Geometry: final body of the model. Coordinates: model frame, mm. A direction names the side the tool comes from. Give positions to 0.01 mm unless a question says otherwise; leave off trailing zeros. Write each loop counter-clockwise with the first axis right and the second up, starting at its lowest first coordinate (ties: lowest second). Pieces come first, ordered by that corner, then holes.
Autodesk Inventor part; units mm, degrees
ref_plane "Work Plane1" through (4.5, 0, 0) normal (1, 0, 0) x (0, 0, -1)
ref_plane "YZ Plane" through (0, 0, 0) normal (1, 0, 0) x (0, 1, 0)
ref_plane "XZ Plane" through (0, 0, 0) normal (0, 1, 0) x (-1, 0, 0)
sketch "Sketch2" plane through (0, 0, 0) normal (1, 0, 0) x (0, 1, 0)
  line L0 (0, 0) -> (0, -3)
  line L1 (13, 0) -> (13, -16)
  arc A0 (13, 0) -> (0, 0) centre (6.5, 0) ccw
  line L2 (-3.1385, 0) -> (18.8309, 0)
  line L3 (0, -52.4723) -> (0, 16.3287)
  line L4 (0, -3) -> (6.5, -9.5)
  line L5 (0, -3) -> (9.1924, -3) construction
  line L6 (6.5, -9.5) -> (6.5, -16)
  line L7 (6.5, -16) -> (0, -22.5)
  line L8 (6.5, -16) -> (15.6924, -16) construction
  line L9 (0, -22.5) -> (0, -27.5)
  line L10 (0, -27.5) -> (6.5, -34)
  line L11 (0, -27.5) -> (9.1924, -27.5) construction
  line L12 (13, -16) -> (13, -34)
  line L13 (13, -34) -> (13, -40.5)
  arc A1 (6.5, -34) -> (13, -40.5) centre (11.1419, -35.8581) ccw
  circle A2 centre (9.75, -38) radius 1.625
  dimension "d4" = 13
  dimension "d9" = 45
  dimension "d10" = 6.5
  dimension "d11" = 3
  dimension "d12" = 6.5
  dimension "d13" = 135
  dimension "d14" = 6.5
  dimension "d15" = 5
  dimension "d16" = 45
  dimension "d17" = 6.5
  dimension "d18" = 18
  dimension "d19" = 6.5
  dimension "d20" = 5
  dimension "d21" = 3.25
  dimension "d22" = 3.25
  dimension "d23" = 2.5
  dimension "d96" = 16
extrude "Extrusion1" add sketch "Sketch2" along normal mid plane 13 contours L2 L1 L12 L13 A1 L10 L3 L7 L6 L4 L0 | A0 L2
sketch "Sketch3" plane through (-6.5, 13, 0) normal (0, 1, 0) x (1, 0, 0)
  line L0 (0, 34) -> (13, 34)
  line L1 (0, 41) -> (1.5, 41)
  line L2 (1.5, 41) -> (1.5, 34)
  line L3 (1.5, 34) -> (0, 34)
  line L4 (0, 34) -> (0, 41)
  line L5 (0, 0) -> (0, 40.5)
  line L6 (3.5, 41) -> (7.5, 41)
  line L7 (7.5, 41) -> (7.5, 34)
  line L8 (7.5, 34) -> (3.5, 34)
  line L9 (3.5, 34) -> (3.5, 41)
  line L10 (9.5, 41) -> (13, 41)
  line L11 (13, 41) -> (13, 34)
  line L12 (13, 34) -> (9.5, 34)
  line L13 (9.5, 34) -> (9.5, 41)
  line L14 (13, 40.5) -> (13, 0)
  point P0 (6.5, 0)
  dimension "d47" = 1.5
  dimension "d48" = 7
  dimension "d49" = 4
  dimension "d50" = 7
  dimension "d51" = 2
  dimension "d52" = 7
  dimension "d53" = 2
extrude "Extrusion2" cut sketch "Sketch3" against normal blind 13
ref_plane "Work Plane1" through (4.5, 0, 0) normal (1, 0, 0) x (0, 0, -1)
sketch "Sketch4" plane through (4.5, 0, 0) normal (1, 0, 0) x (0, 0, -1)
  arc A0 (0, 13) -> (0, 0) centre (0, 6.5) ccw
  line L0 (0, 13) -> (34, 13)
  line L1 (34, 13) -> (34, 6.5)
  line L2 (34, 6.5) -> (27.5, 0)
  line L3 (27.5, 0) -> (22.5, 0)
  line L4 (22.5, 0) -> (16, 6.5)
  line L5 (34, 13) -> (34, 6.5)
  line L6 (34, 6.5) -> (27.5, 0)
  line L7 (27.5, 0) -> (22.5, 0)
  line L8 (22.5, 0) -> (16, 6.5)
  line L9 (16, 6.5) -> (9.5, 6.5)
  line L10 (9.5, 6.5) -> (3, 0)
  line L11 (3, 0) -> (0, 0)
  arc A1 (0, 13) -> (0, 0) centre (0, 6.5) ccw
  line L12 (0, 13) -> (34, 13)
  line L13 (0, 13) -> (0, 2)
  line L14 (0, 2) -> (2, 2)
  line L15 (4, 5) -> (7.5, 8.5)
  line L16 (2.1716, 2) -> (11.364, 2) construction
  line L17 (32, 13) -> (32, 7.3284)
  line L18 (32, 7.3284) -> (26.6716, 2)
  line L19 (32, 7.3284) -> (39.5355, 7.3284) construction
  line L20 (26.6716, 2) -> (23.3284, 2)
  line L21 (23.3284, 2) -> (16.8284, 8.5)
  line L22 (23.3284, 2) -> (32.5208, 2) construction
  line L23 (16.8284, 8.5) -> (7.5, 8.5)
  line L24 (2, 2) -> (2, 13)
  line L25 (0, 13) -> (2, 13)
  line L26 (2.1716, 13) -> (32, 13)
  line L27 (4, 13) -> (4, 5)
  dimension "d57" = 11
  dimension "d59" = 45
  dimension "d60" = 2
  dimension "d62" = 2
  dimension "d63" = 2
  dimension "d64" = 135
  dimension "d65" = 2
  dimension "d66" = 2
  dimension "d67" = 135
  dimension "d94" = 2
  dimension "d97" = 2
  dimension "d98" = 2
  dimension "d99" = 2
extrude "Extrusion3" cut sketch "Sketch4" against normal blind 9 contours L0 L24 L14 L13 | L0 L17 L18 L20 L21 L23 L15 L27
sketch "Sketch6" plane through (1, 13, -34) normal (0, 0, -1) x (-1, 0, 0)
  line L0 (1, -15.6) -> (1, 2.6)
  line L1 (10.1, -13) -> (-8.1, -13)
  circle A0 centre (1, -3) radius 0.75
  line L2 (0, 0) -> (4, 0)
  circle A1 centre (1, -10) radius 0.75
  point P0 (1, -13)
  dimension "d80" = 1.5
  dimension "d81" = 3
  dimension "d82" = 1.5
  dimension "d83" = 3
extrude "Extrusion5" cut sketch "Sketch6" against normal blind 9
sketch "Sketch7" plane through (3, 13, -34) normal (1, 0, 0) x (0, 0, -1)
  line L0 (6.5, 0) -> (0, 0)
  line L1 (6.5, 0) -> (11.5, 0)
  line L2 (11.5, 0) -> (11.5, -2)
  line L3 (11.5, -2) -> (6.5, -2)
  line L4 (6.5, -2) -> (6.5, 0)
  point P0 (-34, -13)
  dimension "d86" = 5
  dimension "d87" = 2
extrude "Extrusion6" add sketch "Sketch7" against normal blind 2
sketch "Sketch8" plane through (-5, 13, -40.5) normal (-1, 0, 0) x (0, 0, 1)
  line L0 (0, 0) -> (6.5, 0)
  line L1 (-5, -2) -> (0, -2)
  line L2 (0, -2) -> (0, 0)
  line L3 (0, 0) -> (-5, 0)
  line L4 (-5, 0) -> (-5, -2)
  point P0 (40.5, -13)
  dimension "d90" = 5
  dimension "d91" = 2
extrude "Extrusion7" add sketch "Sketch8" against normal blind 2
sketch "Sketch9" plane through (4.5, 5, -4) normal (0, 0, -1) x (-1, 0, 0)
  line L0 (0, -3) -> (0, 8)
  line L1 (9, 8) -> (0, 8)
  line L2 (9, 8) -> (9, -3)
  line L3 (0, -3) -> (9, -3)
  circle A0 centre (4.5, 5) radius 0.75
  circle A1 centre (4.5, 1) radius 0.75
  point P0 (4.5, -5)
  dimension "d100" = 1.5
  dimension "d101" = 3
  dimension "d102" = 4.5
  dimension "d103" = 1.5
  dimension "d105" = 4
  dimension "d106" = 4.5
extrude "Extrusion8" cut sketch "Sketch9" against normal blind 2 contours A0 | A1
properties part number "pinkie"
Item 1: Line query: L1, parallel to X at y = 11, z = -31; L2, parallel to Y at x = 0, z = -3.3; L3, parallel to X at y = 7, z = -36. Output: solid intervals per line, ascending.
Found:
L1: x = -6.5 to -4.5, 4.5 to 6.5
L2: y = 0.3 to 5.25, 6.75 to 9.25, 10.75 to 13
L3: x = -5 to -3, 1 to 3
Item 2: Pull-direction query (Y, two-part tool) for faces 1 (the face through (0.098, 10.744, -3.014)), 2 (the face through (1.99, 7, -38.66)), 3 (the face through (4.5, 9, -21)); classes: +Y half, -Y half, draft (parallel to the pull), parting line (faces both ways), or undercut.
Found:
face 1: undercut
face 2: -Y half
face 3: draft
Item 3: Section A-A, the plane y = 3. Return the cut outline in (x, z), plus the area to 3 significant figures.
Found:
outline: (-6.5, -30.5) - (-0.75, -30.5) - (-0.75, -27.67) - (-4.5, -27.67) - (-4.5, -22.33) - (4.5, -22.33) - (4.5, -27.67) - (0.75, -27.67) - (0.75, -30.5) - (6.5, -30.5) - (6.5, -19.5) - (-6.5, -19.5) - close; (-6.5, -6) - (6.5, -6) - (6.5, 5.48) - (-6.5, 5.48) - close; hole (-4.5, -2) - (4.5, -2) - (4.5, 0) - (-4.5, 0) - close
area: 222 mm2
Item 4: Section D-D, the plane z = -15.5. Return the cut outline in (x, y).
Found:
outline: (-6.5, 6.5) - (6.5, 6.5) - (6.5, 13) - (4.5, 13) - (4.5, 8.5) - (-4.5, 8.5) - (-4.5, 13) - (-6.5, 13) - close
Item 5: Section B-B, the plane x = 1.75. Return the cut outline in (y, z) (3 decimals).
Found:
outline: (0, -27.5) - (6.5, -34) arc R5 ccw to (11, -40.856) - (11, -45.5) - (13, -45.5) - (13, -32) - (7.328, -32) - (2, -26.672) - (2, -23.328) - (8.5, -16.828) - (8.5, -7.5) - (5, -4) - (13, -4) - (13, -2) - (2, -2) - (2, 0) - (13, 0) arc R6.5 ccw to (0, 0) - (0, -3) - (6.5, -9.5) - (6.5, -16) - (0, -22.5) - close; hole circle Ø3.25 at (9.75, -38)
Item 6: Pin query (flat end, axial travel): pin 1 Ø7 at (x, y) = (0.5, 6) entering from +Z; pin 2 Ø0.8 at (x, y) = (-6, 10) entering from -Z; pin 3 Ø4.5 at (x, y) = (0.5, 5) entering from -Z; pin 4 Ø2 at (x, y) = (0, 11) entering from +Z. Return the tip coordinate at first contact, or that it passes through.
Found:
pin 1: stops at z = 6.5
pin 2: stops at z = -34
pin 3: stops at z = -38.93
pin 4: stops at z = 5.48
Item 7: Section C-C, the plane z = -38. Return the cut outline in (x, y) (3 decimals), plus the area to 3 significant figures.
Found:
outline: (-5, 6.624) - (-3, 6.624) - (-3, 8.125) - (-5, 8.125) - close; (-5, 11.375) - (-3, 11.375) - (-3, 13) - (-5, 13) - close; (1, 6.624) - (3, 6.624) - (3, 8.125) - (1, 8.125) - close; (1, 11.375) - (3, 11.375) - (3, 13) - (1, 13) - close
area: 12.5 mm2
Item 8: Reachability of faces 4 (the face through (-6, 10, -34)), 5 (the face through (-1, 10, -34)), 6 (the face through (0, 8, 0)) from +Z, -Z, +X, -X, +Y, -Y: full face, straight path, thin tool, end or side. Return the list, or none.
Found:
face 4: -Z, -X, +Y, -Y
face 5: -Z, +Y, -Y
face 6: +Y
